Autodesk Inventor part; units mm, degrees
ref_plane "YZ Plane" through (0, 0, 0) normal (1, 0, 0) x (0, 1, 0)
ref_plane "XZ Plane" through (0, 0, 0) normal (0, 1, 0) x (-1, 0, 0)
ref_plane "XY Plane" through (0, 0, 0) normal (0, 0, 1) x (1, 0, 0)
sketch "Boceto1" plane through (0, 0, 0) normal (0, 1, 0) x (-1, 0, 0)
  circle A0 centre (0, 0) radius 62.75
  circle A1 centre (0, 0) radius 64.5
  circle A2 centre (0, 0) radius 58.85
  circle A3 centre (0, 0) radius 62.75
  circle A4 centre (0, 0) radius 58.85
  dimension "d0" = 125.5
  dimension "d1" = 129
  dimension "d2" = 117.7
extrude "Extrusión1" add sketch "Boceto1" along normal blind 5
sketch "Boceto3" plane through (0, 0, 0) normal (0, -1, 0) x (1, 0, 0)
  circle A0 centre (0, 0) radius 58.85
  circle A1 centre (0, 0) radius 62.75
extrude "Extrusión2" add sketch "Boceto3" against normal blind 3
sketch "Boceto4" plane through (0, 0, 0) normal (0, -1, 0) x (1, 0, 0)
  line L0 (-7.5, 12.5) -> (7.5, 12.5)
  line L1 (7.5, 12.5) -> (7.5, -12.5)
  line L2 (7.5, -12.5) -> (-7.5, -12.5)
  line L3 (-7.5, -12.5) -> (-7.5, 12.5)
  line L4 (-7.5, 12.5) -> (7.5, -12.5) construction
  line L5 (7.5, 12.5) -> (-7.5, -12.5) construction
  point P0 (0, 0)
  dimension "d7" = 15
  dimension "d8" = 25
extrude "Extrusión3" add sketch "Boceto4" along normal blind 5
sketch "Boceto5" plane through (-7.5, 0, -12.5) normal (-1, 0, 0) x (0, 0, 1)
  line L0 (0, -5) -> (25, -5)
  line L1 (25, -5) -> (25, 0)
  line L2 (25, 0) -> (27, 0)
  line L3 (77, 0) -> (-52, 0)
  line L4 (27, 0) -> (25, -5)
  line L5 (0, 0) -> (-2, 0)
  line L6 (-2, 0) -> (0, -5)
  line L7 (0, 0) -> (0, -5)
  point P0 (12.5, 0)
  dimension "d11" = 2
  dimension "d12" = 2
extrude "Extrusión4" add sketch "Boceto5" against normal blind 15 contours L6 L3 L7 | L1 L2 L4
sketch "Boceto9" plane through (0, 5, 0) normal (0, 1, 0) x (1, 0, 0)
  line L0 (-7.5, 12.5) -> (7.5, 12.5)
  line L1 (7.5, 12.5) -> (7.5, -12.5)
  line L2 (7.5, -12.5) -> (-7.5, -12.5)
  line L3 (-7.5, -12.5) -> (-7.5, 12.5)
  line L4 (-7.5, 12.5) -> (7.5, -12.5) construction
  line L5 (7.5, 12.5) -> (-7.5, -12.5) construction
  point P0 (0, 0)
  dimension "d15" = 25
  dimension "d16" = 15
extrude "Extrusión5" cut sketch "Boceto9" against normal blind 4
sketch "Boceto10" plane through (0, 1, 0) normal (0, 1, 0) x (1, 0, 0)
  circle A0 centre (0, -7) radius 1.5875
  circle A1 centre (0, 7) radius 1.5875
  point P0 (0, 0)
  dimension "d19" = 3.175
  dimension "d20" = 3.175
  dimension "d21" = 14
  dimension "d22" = 7
extrude "Extrusión6" cut sketch "Boceto10" against normal blind 6
properties part number "Base_Taza"
Could you check a few things on this model? Use its own coordinates, in mm. A direction names the side the tool comes from. Round coordinates to 2 decimals unless told otherwise and drop trailing zeros. Loops run counter-clockwise (first coordinate to the right, second up) from the corner with the lowest first, then second, coordinate; pieces in that order, holes last. Notation, with made-up numbers: M 67,-27.5 L 126,-27.5 A25 cw 126,-10.5 Z; hole C -14.5,52 d9. An arc over 180 degrees is marked long. Write item = value, one per line.
1. I need wall thicknesses on probe 1 along X at (y, z) = (-0.85, -7); probe 2 along Z at (x, y) = (0, -2.15); probe 3 along Z at (x, y) = (-22, 4). Which ranges of each line are inside material? Lowest first, please.
Results below:
probe_1 = -7.5 to -1.59, 1.59 to 7.5
probe_2 = -13.64 to -8.59, -5.41 to 5.41, 8.59 to 13.64
probe_3 = -60.63 to -58.77, -54.58 to 54.58, 58.77 to 60.63
2. I want a section at D-D, the plane x = 26. Write out the boundary of the cut face in (y, z).
Results below:
outline = M 0,-59.03 L 5,-59.03 L 5,-57.11 L 3,-57.11 L 3,-52.8 L 5,-52.8 L 5,52.8 L 3,52.8 L 3,57.11 L 5,57.11 L 5,59.03 L 0,59.03 Z
3. Thinking about a two-plate mould opening in Z: for faces 1 (the face through (-7.5, 3, 0)), 2 (the face through (-0.1, -2.5, 13.5)), 3 (the face through (13, 0, 1)), 4 (the face through (0, 3, 12.5)), which applies, +Z half, -Z half, draft (parallel to the pull), parting line (faces both ways), or undercut?
Results below:
face_1 = undercut
face_2 = +Z half
face_3 = draft
face_4 = undercut
4. Will these pins go through, and if not, where does the flat tip stop? P1, Ø12, axis at x = 15.5, z = -11, coming from the -Y side; P2, Ø4, axis at x = 0, z = 7, coming from the -Y side; P3, Ø2.5, axis at y = -3.5, z = -7, coming from the -X side; P4, Ø1.2, axis at y = 2.5, z = -6, coming from the -X side.
Results below:
P1 = 0
P2 = -5
P3 = -7.5
P4 = -64.27
5. Which directions (+Z, -Z, +X, -X, +Y, -Y) give clear straight access to the entire face, cutting with the end or side of a thin tool? Please do faces 5 (the face through (7.5, 3, 0)), 6 (the face through (7.5, -2, 0)), 7 (the face through (-7.5, -2, 0)), 8 (the face through (-61.522, 2.465, -19.374)).
Results below:
face_5 = +Y
face_6 = +Z, -Z, +X, -Y
face_7 = +Z, -Z, -X, -Y
face_8 = +Y, -Y
6. I want a section at A-A, the plane x = 0. Write out the boundary of the cut face in (y, z).
Results below:
outline = M -5,-12.5 L 0,-14.5 L 0,-64.5 L 5,-64.5 L 5,-62.75 L 3,-62.75 L 3,-58.85 L 5,-58.85 L 5,-12.5 L 1,-12.5 L 1,-8.59 L -5,-8.59 Z; M -5,-5.41 L 1,-5.41 L 1,5.41 L -5,5.41 Z; M -5,8.59 L 1,8.59 L 1,12.5 L 5,12.5 L 5,58.85 L 3,58.85 L 3,62.75 L 5,62.75 L 5,64.5 L 0,64.5 L 0,14.5 L -5,12.5 Z
7. I want a section at C-C, the plane z = -7. Write out the boundary of the cut face in (x, y).
Results below:
outline = M -64.12,0 L -7.5,0 L -7.5,-5 L -1.59,-5 L -1.59,1 L -7.5,1 L -7.5,5 L -58.43,5 L -58.43,3 L -62.36,3 L -62.36,5 L -64.12,5 Z; M 1.59,-5 L 7.5,-5 L 7.5,0 L 64.12,0 L 64.12,5 L 62.36,5 L 62.36,3 L 58.43,3 L 58.43,5 L 7.5,5 L 7.5,1 L 1.59,1 Z
8. I want a section at B-B, the plane y = -3.25. Write out the boundary of the cut face in (x, z) (1 decimal).
Results below:
outline = M -7.5,-13.2 L 7.5,-13.2 L 7.5,13.2 L -7.5,13.2 Z; hole C 0,-7 d3.2; hole C 0,7 d3.2
